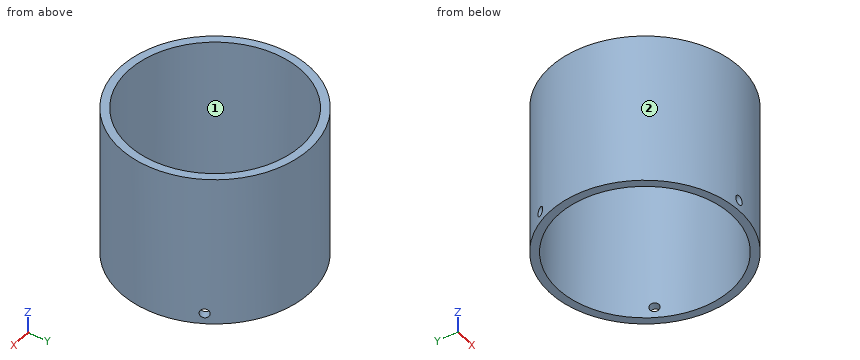
```python
from build123d import *

# Parameters (mm, degrees)
ESQUISSE1_R                  = 35
ESQUISSE1_R_2                = 32
BASE_EXTRUSION_DEPTH         = 56
ESQUISSE2_R                  = 1.7
ENL_V_MAT_EXTRU_1_DEPTH      = 36
R_P_TITION_CIRCULAIRE1_COUNT = 3


with BuildPart() as part:
    # Esquisse1 → Base-Extrusion (new body)
    with BuildSketch(Plane.XY):
        Circle(ESQUISSE1_R)
        Circle(ESQUISSE1_R_2, mode=Mode.SUBTRACT)
    extrude(amount=BASE_EXTRUSION_DEPTH)

    # Esquisse2 → Enlèv. mat.-Extru.1 (cut, through all)
    with BuildSketch(Plane(origin=(0, 0, 0), x_dir=(1, 0, 0), z_dir=(0, 1, 0))):
        with Locations((0, -4)):
            Circle(ESQUISSE2_R)
    enl_v_mat_extru_1 = extrude(amount=-ENL_V_MAT_EXTRU_1_DEPTH, mode=Mode.SUBTRACT)

    # Répétition circulaire1: Enlèv. mat.-Extru.1 ×3 about axis
    r_p_tition_circulaire1_axis = Axis((0, 0, 0), (0, 0, -1))
    for i in range(1, R_P_TITION_CIRCULAIRE1_COUNT):
        add(enl_v_mat_extru_1.rotate(r_p_tition_circulaire1_axis, i * 360 / R_P_TITION_CIRCULAIRE1_COUNT), mode=Mode.SUBTRACT)


solid = part.part
```
Here's how the part is built. I have some questions about the finished solid (model axes, mm). Face numbers are marked on the shaded views. Round coordinates to 2 decimals unless told otherwise and drop trailing zeros. Write each loop counter-clockwise with the first axis right and the second up, starting at its lowest first coordinate (ties: lowest second). Pieces come first, ordered by that corner, then holes. Notation, with made-up numbers: M 83.5,-33 L 96.5,-33 A19 ccw 96.5,-2 Z; hole C 48.5,62.5 d7. An arc over 180 degrees is marked long. Answer as CSV lines item,"result". Start each with the question number.
1. Suppose I cut it at C-C on x = 15.5. Write out the boundary of the cut face in (y, z).
2. Suppose I cut it at B-B on y = 0. Write out the boundary of the cut face in (x, z), then the cut area to 3 significant figures.
3. Suppose I cut it at A-A on x = 0. Write out the boundary of the cut face in (y, z).
4. Suppose I cut it at D-D on z = 15. Write out the boundary of the cut face in (x, y), then the cut area to 3 significant figures.
5. I'm going to push flat-ended pins straight in: pin 1 Ø1.5 at (x, z) = (-12, 6.5) entering from +Y; pin 2 Ø12 at (y, z) = (-25.5, 6.5) entering from -X; pin 3 Ø12 at (x, y) = (-23, 4.5) entering from +Z; pin 4 Ø2 at (x, z) = (23.5, 23.5) entering from -Y. Where does each tip first touch, or does it pass through?
6. I need wall thicknesses on probe 1 along Y at (x, z) = (0, 21); probe 2 along Z at (x, y) = (0, -33.3); probe 3 along Y at (x, z) = (-6, 32.5). Which ranges of each line are inside material? Lowest first, please.
7. Thinking about a two-plate mould opening in Y: for the marked faces 1 and 2, which applies, released by +Y, released by -Y, zero draft, split by the parting line, or undercut?
Check result:
1,outline,"M -31.38,0 L -28,0 L -28,56 L -31.38,56 Z; M 28,0 L 31.38,0 L 31.38,56 L 28,56 Z"
2,outline,"M -35,0 L -32,0 L -32,56 L -35,56 Z; M 32,0 L 35,0 L 35,56 L 32,56 Z"
2,area,"336 mm2"
3,outline,"M -35,0 L -32,0 L -32,2.3 L -35,2.3 Z; M -35,5.7 L -32,5.7 L -32,56 L -35,56 Z; M 32,0 L 35,0 L 35,56 L 32,56 Z"
4,outline,"C 0,0 d70; hole C 0,0 d64"
4,area,"631 mm2"
5,pin 1,"stops at y = 33.14"
5,pin 2,"stops at x = -29.06"
5,pin 3,"passes through"
5,pin 4,"stops at y = -26.81"
6,probe 1,"y = -35 to -32, 32 to 35"
6,probe 2,"z = 0 to 2.3, 5.7 to 56"
6,probe 3,"y = -34.48 to -31.43, 31.43 to 34.48"
7,face 1,"undercut"
7,face 2,"split by the parting line"
